For this review, take the finished solid that the model builds, in its own axes (mm). A direction names the side the tool comes from. Round coordinates to 2 decimals unless told otherwise and drop trailing zeros. Order: outer loops, then holes, each group sorted by start corner. A loop starts at its lowest first (then second) coordinate and runs counter-clockwise, first axis right, second up.
```python
from build123d import *

# Parameters (mm, degrees)
BOSS_EXTRU_1_DEPTH      = 5
D_GAGEMENT_M31_D        = 3.6
ENL_V_MAT_EXTRU_2_DEPTH = 10


with BuildPart() as part:
    # Esquisse1 → Boss.-Extru.1 (new body)
    with BuildSketch(Plane(origin=(0, 0, 0), x_dir=(1, 0, 0), z_dir=(0, 1, 0))):
        Polygon((-20, -23.663326483), (-32.5, -45.313961578), (-137.5, -227.179296373), (-150, -248.829931467), (-130, -283.470947619), (-105, -283.470947619), (105, -283.470947619), (130, -283.470947619), (150, -248.829931467), (137.5, -227.179296373), (32.5, -45.313961578), (20, -23.663326483), align=None)
        with BuildLine():
            ThreePointArc((-96.494247139, -272.786646223), (-100.288342364, -273.286148335), (-103.324374158, -270.956519204))
            Line((-103.324374158, -270.956519204), (-125.824374158, -231.985376033))
            ThreePointArc((-125.824374158, -231.985376033), (-126.32387627, -228.191280808), (-123.994247139, -225.155249015))
            Line((-123.994247139, -225.155249015), (-102.343612044, -212.655249015))
            ThreePointArc((-102.343612044, -212.655249015), (-98.549516819, -212.155746902), (-95.513485025, -214.485376033))
            Line((-95.513485025, -214.485376033), (-73.013485025, -253.456519204))
            ThreePointArc((-73.013485025, -253.456519204), (-72.513982913, -257.250614429), (-74.843612044, -260.286646223))
            Line((-74.843612044, -260.286646223), (-96.494247139, -272.786646223))
        make_face(mode=Mode.SUBTRACT)
        with BuildLine():
            ThreePointArc((74.843612044, -260.286646223), (72.513982913, -257.250614429), (73.013485025, -253.456519204))
            Line((73.013485025, -253.456519204), (95.513485025, -214.485376033))
            ThreePointArc((95.513485025, -214.485376033), (98.549516819, -212.155746902), (102.343612044, -212.655249015))
            Line((102.343612044, -212.655249015), (123.994247139, -225.155249015))
            ThreePointArc((123.994247139, -225.155249015), (126.32387627, -228.191280808), (125.824374158, -231.985376033))
            Line((125.824374158, -231.985376033), (103.324374158, -270.956519204))
            ThreePointArc((103.324374158, -270.956519204), (100.288342364, -273.286148335), (96.494247139, -272.786646223))
            Line((96.494247139, -272.786646223), (74.843612044, -260.286646223))
        make_face(mode=Mode.SUBTRACT)
        with BuildLine():
            Line((22.5, -89.022310332), (-22.5, -89.022310332))
            ThreePointArc((-22.5, -89.022310332), (-26.035533906, -87.557844238), (-27.5, -84.022310332))
            Line((-27.5, -84.022310332), (-27.5, -59.022310332))
            ThreePointArc((-27.5, -59.022310332), (-26.035533906, -55.486776426), (-22.5, -54.022310332))
            Line((-22.5, -54.022310332), (22.5, -54.022310332))
            ThreePointArc((22.5, -54.022310332), (26.035533906, -55.486776426), (27.5, -59.022310332))
            Line((27.5, -59.022310332), (27.5, -84.022310332))
            ThreePointArc((27.5, -84.022310332), (26.035533906, -87.557844238), (22.5, -89.022310332))
        make_face(mode=Mode.SUBTRACT)
    extrude(amount=BOSS_EXTRU_1_DEPTH)

    # Dégagement M31 (through all)
    with Locations(Plane(origin=(-143.169872981, 5, 246.999804448), x_dir=(0, 0, 1), z_dir=(0, 1, 0))):
        with Locations((0, 0), (31.471143171, 18.169872981), (31.471143171, 268.169872981), (0, 286.339745962), (-216.506350946, 125), (-216.506350946, 161.339745962)):
            Hole(D_GAGEMENT_M31_D / 2)

    # Esquisse6 → Enlèv. mat.-Extru.2 (cut)
    with BuildSketch(Plane(origin=(0, 0, 0), x_dir=(-1, 0, 0), z_dir=(0, -1, 0))):
        with BuildLine():
            Line((-16.437822174, -183.172945427), (-6.062177826, -201.144088597))
            ThreePointArc((-6.062177826, -201.144088597), (0, -204.644088597), (6.062177826, -201.144088597))
            Line((6.062177826, -201.144088597), (16.437822174, -183.172945427))
            ThreePointArc((16.437822174, -183.172945427), (16.437822174, -176.172945427), (10.375644347, -172.672945427))
            Line((10.375644347, -172.672945427), (-10.375644347, -172.672945427))
            ThreePointArc((-10.375644347, -172.672945427), (-16.437822174, -176.172945427), (-16.437822174, -183.172945427))
        make_face()
    extrude(amount=-ENL_V_MAT_EXTRU_2_DEPTH, mode=Mode.SUBTRACT)


solid = part.part
```
Q1. Take a section at B-B, the plane z = 265. State the section outline as (x, y) points.
Q2. Take a section at D-D, the plane y = 2.9. Count the separate pieces of the cut face and the enclosed holes in it, plus the area to 3 significant figures.
Q3. Take a section at A-A, the plane x = 89. State the section outline as (y, z) points.
Q4. Mouldability with a two-part tool opening along Z and no side actions: class faces 3 (the face through (-140.14, 2.46, 265.91)), 4 (the face through (-11.18, 2.46, 192.28)), 5 (the face through (-2, 5, 209)) as +Z half, -Z half, draft (parallel to the pull), parting line (faces both ways), or undercut.
Q5. Wall thickness on line 1 (X direction, y = 0.45, z = 217.5); line 2 (X direction, y = 1.95, z = 268.5); line 3 (Z direction, x = -124.5, y = 4.25): over which ranges is each line inside the solid? List them lowest first.
Q6. Clearance check with flat-ended pins moving along their axes: pin 1 (2.5 mm diameter, centred on y = 2, z = 66, fed in from -X); pin 2 (2.5 mm diameter, centred on y = 3, z = 69, fed in from +X). State where each tip first meets the part, or that it passes through.
Q7. Tool access review of faces 1 (the face through (-2, 0, 209)), 2 (the face through (16.386, 2.465, 176.084)): name each direction out of +Z, -Z, +X, -X, +Y, -Y from which nothing blocks a thin tool from reaching the whole face with its end or side.
Q8. Take a section at C-C, the plane z = 80.5. State the section outline as (x, y) points, plus the area to 3 significant figures.
Working result:
1. outline: (-140.66, 0) - (-106.76, 0) - (-106.76, 5) - (-140.66, 5) - close; (-83.01, 0) - (83.01, 0) - (83.01, 5) - (-83.01, 5) - close; (106.76, 0) - (140.66, 0) - (140.66, 5) - (106.76, 5) - close
2. separate pieces: 1
2. enclosed holes: 10
2. area: 41,400 mm2
3. outline: (0, 143.17) - (5, 143.17) - (5, 225.77) - (0, 225.77) - close; (0, 268.46) - (5, 268.46) - (5, 283.47) - (0, 283.47) - close
4. face 3: +Z half
4. face 4: undercut
4. face 5: draft
5. line 1: x = -131.91 to -110.73, -93.77 to 93.77, 110.73 to 131.91
5. line 2: x = -138.64 to -104.74, -89.07 to 89.07, 104.74 to 138.64
5. line 3: z = 204.66 to 225.49, 234.28 to 276.74, 280.2 to 283.47
6. pin 1: stops at x = -45.16
6. pin 2: stops at x = 46.9
7. face 1: +Z, -Z, +X, -X, -Y
7. face 2: +Y, -Y
8. outline: (-52.81, 0) - (-27.5, 0) - (-27.5, 5) - (-52.81, 5) - close; (27.5, 0) - (52.81, 0) - (52.81, 5) - (27.5, 5) - close
8. area: 253 mm2
